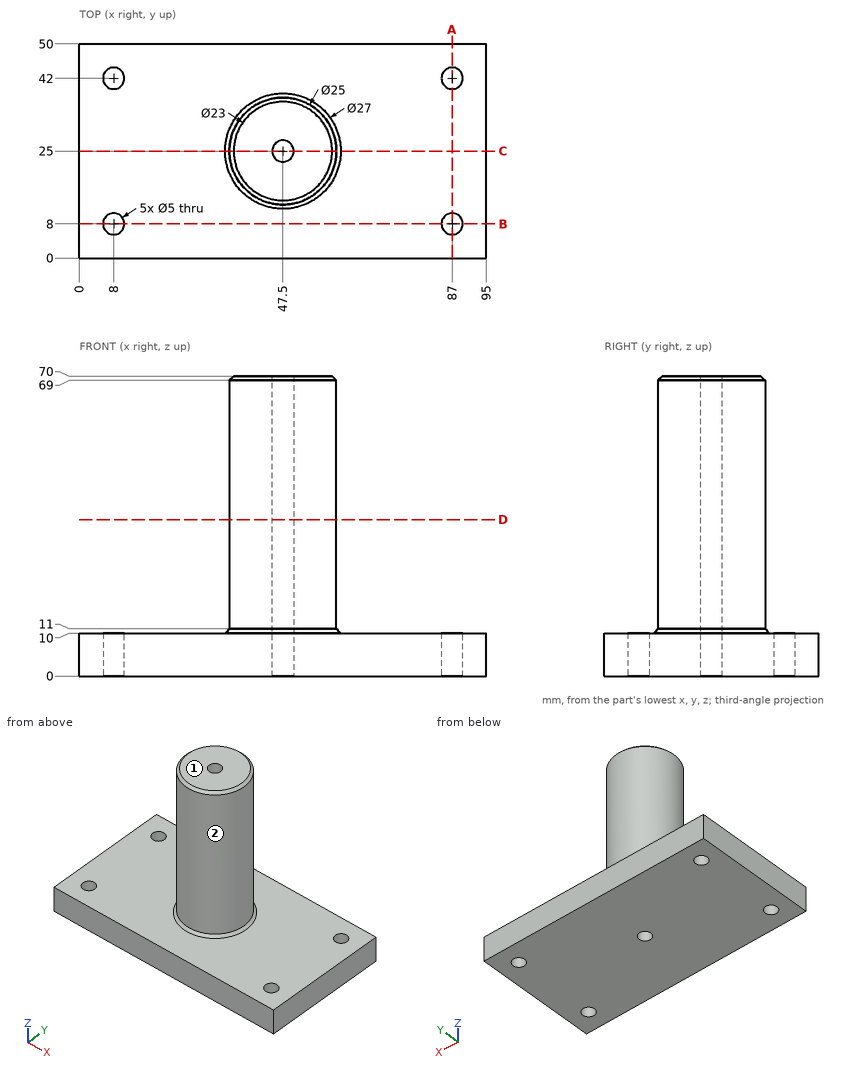
Geometry: see drawing. Coordinates: mm, zero at the bounding-box minimum. A direction names the side the tool comes from. Round coordinates to 2 decimals unless told otherwise and drop trailing zeros. Order: outer loops, then holes, each group sorted by start corner. A loop starts at its lowest first (then second) coordinate and runs counter-clockwise, first axis right, second up. Notation, with made-up numbers: (64.25, 78.5) - (117.25, 78.5) arc R26 cw to (117.25, 115.5) - close; hole circle Ø3 at (40.25, 12.5). An arc over 180 degrees is marked (long way). One line per question, with ' | ' between items. Start each with the question number.
1) Set-up query: the marked faces 1 and 2. Return all of +Z, -Z, +X, -X, +Y, -Y with unobstructed straight access to the full face (end or side cutting, diameter ignored); none if empty.
2) Contact query for flat-ended pins moving along their axis: P1, Ø1, axis at x = 59.5, y = 5, coming from the +Z side; P2, Ø12, axis at y = 11, z = 52.5, coming from the +X side; P3, Ø12, axis at x = 45, z = 55, coming from the -Y side. Output: stop coordinate, or through.
3) Cut plane D-D, the plane z = 36.5. Return the cut outline in (x, y).
4) Cut plane A-A, the plane x = 87. Return the cut outline in (y, z).
5) Ray query, probe 1 along Y at (x, z) = (87, 3); probe 2 along Z at (x, y) = (29.5, 18); probe 3 along X at (y, z) = (19.5, 11). Return the intervals inside material, ascending.
6) Cut plane B-B, the plane y = 8. Return the cut outline in (x, z), then the cut area to 3 significant figures.
7) Cut plane C-C, the plane y = 25. Return the cut outline in (x, z).
Worked out:
1) face 1: +Z, +X, -X, +Y, -Y | face 2: +Z
2) P1: stops at z = 10 | P2: stops at x = 57.1 | P3: stops at y = 12.5
3) outline: circle Ø25 at (47.5, 25); hole circle Ø5 at (47.5, 25)
4) outline: (0, 0) - (5.5, 0) - (5.5, 10) - (0, 10) - close; (10.5, 0) - (39.5, 0) - (39.5, 10) - (10.5, 10) - close; (44.5, 0) - (50, 0) - (50, 10) - (44.5, 10) - close
5) probe 1: y = 0 to 5.5, 10.5 to 39.5, 44.5 to 50 | probe 2: z = 0 to 10 | probe 3: x = 36.28 to 58.72
6) outline: (0, 0) - (5.5, 0) - (5.5, 10) - (0, 10) - close; (10.5, 0) - (84.5, 0) - (84.5, 10) - (10.5, 10) - close; (89.5, 0) - (95, 0) - (95, 10) - (89.5, 10) - close | area: 850 mm^2
7) outline: (0, 0) - (45, 0) - (45, 70) - (36, 70) - (35, 69) - (35, 11) - (34, 10) - (0, 10) - close; (50, 0) - (95, 0) - (95, 10) - (61, 10) - (60, 11) - (60, 69) - (59, 70) - (50, 70) - close
